```python
from build123d import *

# Parameters (mm, degrees)
SKETCH1_W           = 700
SKETCH1_H           = 700
BOSS_EXTRUDE1_DEPTH = 300
SKETCH2_W           = 500
SKETCH2_H           = 500
SKETCH3_W           = 500
SKETCH3_H           = 500
BOSS_EXTRUDE2_DEPTH = 100
SHELL1_T            = -10


with BuildPart() as part:
    # Sketch1 → Boss-Extrude1 (new body)
    with BuildSketch(Plane(origin=(0, 0, 0), x_dir=(1, 0, 0), z_dir=(0, 1, 0))):
        Rectangle(SKETCH1_W, SKETCH1_H)
    extrude(amount=BOSS_EXTRUDE1_DEPTH)

    # Sketch2 → section 1 of loft1
    with BuildSketch(Plane(origin=(0, -250, 0), x_dir=(-1, 0, 0), z_dir=(0, -1, 0)), mode=Mode.PRIVATE) as loft1_s1:
        Rectangle(SKETCH2_W, SKETCH2_H)
    # loft from a face of the part (loft1)
    loft([part.faces().sort_by_distance((0, 0, 0))[0], loft1_s1.sketch])

    # Sketch3 → Boss-Extrude2 (add)
    with BuildSketch(Plane.XZ.offset(250)):
        Rectangle(SKETCH3_W, SKETCH3_H)
    extrude(amount=BOSS_EXTRUDE2_DEPTH)

    # Shell1
    shell1_openings = [part.faces().sort_by_distance(p)[0] for p in [
        (0, 300, 0),
        (0, -350, 0),
    ]]
    offset(amount=SHELL1_T, openings=shell1_openings, kind=Kind.INTERSECTION)


solid = part.part
```
Check sheet for the modelled part. Datum: model origin and axes. Units: mm. A direction names the side the tool comes from. Coordinates: 2 decimals unless noted, no trailing zeros. Order: outer loops, then holes, each group sorted by start corner. A loop starts at its lowest first (then second) coordinate and runs counter-clockwise, first axis right, second up. Notation, with made-up numbers: M 20,17 L 36,17 A33 ccw 36,51 Z; hole C -40,-23.5 d11. An arc over 180 degrees is marked long. Write each question's results on one line, items separated by ' | '. Start each with the question number.
1. Mould release check, pull along Z, two halves, no side actions. Record for faces 6 (the face through (-3, -299, 250)), 7 (the face through (-350, 148, 5)), 8 (the face through (-289.3, -124.82, -4.76)), 9 (the face through (-5, 149, -340)): +Z half, -Z half, draft (parallel to the pull), parting line (faces both ways), or undercut.
2. Cross-section at A-A on y = 26. Record the cut outline in (x, z).
3. Material ranges on probe 1 along Z at (x, y) = (-180.5, 100.5); probe 2 along X at (y, z) = (-10, 320), recorded low to high.
4. Access from +Z, -Z, +X, -X, +Y, -Y to the whole of each face (thin tool, end or side, straight path). Record for faces 1 (the face through (-3, -298, -240)), 2 (the face through (-250, -299, -3)), 3 (the face through (350, 148, 5)), 4 (the face through (-340, 149, 5)), 5 (the face through (-3, -299, -250)).
Checks:
1) face 6: +Z half | face 7: draft | face 8: undercut | face 9: undercut
2) outline: M -350,-350 L 350,-350 L 350,350 L -350,350 Z; hole M -340,-340 L 340,-340 L 340,340 L -340,340 Z
3) probe 1: z = -350 to -340, 340 to 350 | probe 2: x = -346 to -335.23, 335.23 to 346
4) face 1: +Y, -Y | face 2: +Z, -Z, -X, -Y | face 3: +Z, -Z, +X, +Y, -Y | face 4: +Y | face 5: -Z, +X, -X, -Y
